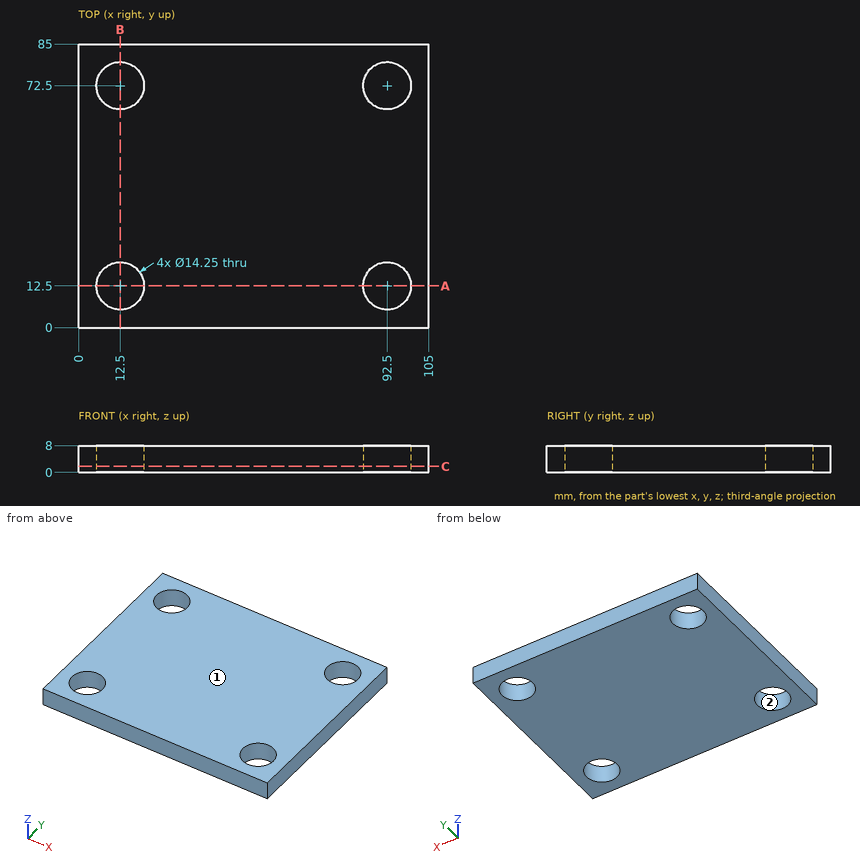
The figure shows three views and two pictorial views of one solid part (mm, origin at its lowest corner). Answer the questions. Round coordinates to 2 decimals unless told otherwise and drop trailing zeros. Write each loop counter-clockwise with the first axis right and the second up, starting at its lowest first coordinate (ties: lowest second). Pieces come first, ordered by that corner, then holes. Notation, with made-up numbers: (65.5, 71) - (117.5, 71) arc R17 cw to (117.5, 88) - close; hole circle Ø2 at (88.25, -37.5). An arc over 180 degrees is marked (long way). Answer in a Markdown table with one row per item. Add a question column.
1. The mould has two halves that part along X. Classify the marked faces 1 and 2: +X half, -X half, draft (parallel to the pull), parting line (faces both ways), or undercut.
2. A cutting plane is placed at A-A, the plane y = 12.5. Determine the outline of the cut face in (x, z) (3 decimals).
3. A cutting plane is placed at C-C, the plane z = 1.75. Determine the outline of the cut face in (x, y) (3 decimals), and give its area (3 significant figures).
4. Find the intervals of material crossed by line 1 along X through (y, z) = (12.5, 3.5) (3 decimals); line 2 along Y through (x, z) = (12.5, 2.75) (3 decimals); line 3 along X through (y, z) = (9, 1), in increasing order. Write a range as from..to.
5. A cutting plane is placed at B-B, the plane x = 12.5. Determine the outline of the cut face in (y, z) (3 decimals).
6. Given pin 1 (8.5 mm diameter, centred on x = 92.5, y = 12.5, fed in from -Z), flat-ended and moving along its own axis, determine where the tip first touches the part or whether it passes through.
Worked out:
| question | item | result |
|---|---|---|
| 1 | face 1 | draft |
| 1 | face 2 | undercut |
| 2 | outline | (0, 0) - (5.375, 0) - (5.375, 8) - (0, 8) - close; (19.625, 0) - (85.375, 0) - (85.375, 8) - (19.625, 8) - close; (99.625, 0) - (105, 0) - (105, 8) - (99.625, 8) - close |
| 3 | outline | (0, 0) - (105, 0) - (105, 85) - (0, 85) - close; hole circle Ø14.25 at (12.5, 12.5); hole circle Ø14.25 at (12.5, 72.5); hole circle Ø14.25 at (92.5, 12.5); hole circle Ø14.25 at (92.5, 72.5) |
| 3 | area | 8,290 mm^2 |
| 4 | line 1 | 0..5.375, 19.625..85.375, 99.625..105 |
| 4 | line 2 | 0..5.375, 19.625..65.375, 79.625..85 |
| 4 | line 3 | 0..6.29, 18.71..86.29, 98.71..105 |
| 5 | outline | (0, 0) - (5.375, 0) - (5.375, 8) - (0, 8) - close; (19.625, 0) - (65.375, 0) - (65.375, 8) - (19.625, 8) - close; (79.625, 0) - (85, 0) - (85, 8) - (79.625, 8) - close |
| 6 | pin 1 | through |
